```python
from build123d import *

# Parameters (mm, degrees)
BOSS_EXTRUDE1_DEPTH                   = 5
TAP_DRILL_FOR_M5X0_8_TAP1_D           = 4.2
TAP_DRILL_FOR_M5X0_8_TAP1_CSINK_D     = 4.25
TAP_DRILL_FOR_M5X0_8_TAP1_CSINK_ANGLE = 90
SKETCH4_W                             = 5
SKETCH4_H                             = 15
SKETCH4_H_2                           = 5
SKETCH4_W_2                           = 15
BOSS_EXTRUDE2_DEPTH                   = 15
TAP_DRILL_FOR_M5X0_8_TAP2_D           = 4.2
TAP_DRILL_FOR_M5X0_8_TAP2_CSINK_D     = 4.25
TAP_DRILL_FOR_M5X0_8_TAP2_CSINK_ANGLE = 90
TAP_DRILL_FOR_M5X0_8_TAP3_D           = 4.2
TAP_DRILL_FOR_M5X0_8_TAP3_CSINK_D     = 4.25
TAP_DRILL_FOR_M5X0_8_TAP3_CSINK_ANGLE = 90
CHAMFER1_SIZE                         = 5


with BuildPart() as part:
    # Sketch1 → Boss-Extrude1 (new body)
    with BuildSketch(Plane(origin=(0, 0, 0), x_dir=(1, 0, 0), z_dir=(0, 1, 0))):
        Polygon((9.5, 0), (20, 0), (20, 20), (0, 20), (0, 0), align=None)
    extrude(amount=BOSS_EXTRUDE1_DEPTH)

    # Tap Drill for M5x0.8 Tap1 (through all)
    with Locations(Plane(origin=(0, 0, 0), x_dir=(-1, 0, 0), z_dir=(0, -1, 0))):
        with Locations((-9.5, 10.5)):
            CounterSinkHole(TAP_DRILL_FOR_M5X0_8_TAP1_D / 2, TAP_DRILL_FOR_M5X0_8_TAP1_CSINK_D / 2, counter_sink_angle=TAP_DRILL_FOR_M5X0_8_TAP1_CSINK_ANGLE)

    # Sketch4 → Boss-Extrude2 (add)
    with BuildSketch(Plane(origin=(0, 5, 0), x_dir=(1, 0, 0), z_dir=(0, 1, 0))):
        with Locations((17.5, 12.5)):
            Rectangle(SKETCH4_W, SKETCH4_H)
        with Locations((17.5, 2.5)):
            Rectangle(SKETCH4_W, SKETCH4_H_2)
        with Locations((7.5, 2.5)):
            Rectangle(SKETCH4_W_2, SKETCH4_H_2)
    extrude(amount=BOSS_EXTRUDE2_DEPTH)

    # Tap Drill for M5x0.8 Tap2 (through all)
    with Locations(Plane.XY):
        with Locations((9.5, 10.5)):
            CounterSinkHole(TAP_DRILL_FOR_M5X0_8_TAP2_D / 2, TAP_DRILL_FOR_M5X0_8_TAP2_CSINK_D / 2, counter_sink_angle=TAP_DRILL_FOR_M5X0_8_TAP2_CSINK_ANGLE)

    # Tap Drill for M5x0.8 Tap3 (through all)
    with Locations(Plane(origin=(20, 0, 0), x_dir=(0, 0, -1), z_dir=(1, 0, 0))):
        with Locations((10.5, 10.5)):
            CounterSinkHole(TAP_DRILL_FOR_M5X0_8_TAP3_D / 2, TAP_DRILL_FOR_M5X0_8_TAP3_CSINK_D / 2, counter_sink_angle=TAP_DRILL_FOR_M5X0_8_TAP3_CSINK_ANGLE)

    # Chamfer1
    chamfer1_edges = [part.edges().sort_by_distance(p)[0] for p in [
        (0, 20, -2.5),
        (17.5, 20, -20),
        (0, 2.5, -20),
    ]]
    chamfer(chamfer1_edges, length=CHAMFER1_SIZE)


solid = part.part
```
The listing builds one solid part. Answer for the finished solid, in the listing's coordinates (mm). A direction names the side the tool comes from. Give positions to 0.01 mm unless a question says otherwise; leave off trailing zeros. Write each loop counter-clockwise with the first axis right and the second up, starting at its lowest first coordinate (ties: lowest second). Pieces come first, ordered by that corner, then holes. Notation, with made-up numbers: (77, 75.25) -> (132, 75.25) arc R25 cw to (132, 89.25) -> close; hole circle Ø4 at (23.25, -24). An arc over 180 degrees is marked (long way). Use one line per item in the form item = value.
1) Each of these flat-tipped pins is pushed along its axis until it touches: P1, Ø1.5, axis at y = 15.5, z = -6.5, coming from the -X side; P2, Ø5, axis at x = 12, y = 16.5, coming from the -Z side; P3, Ø12, axis at y = 11, z = -8.5, coming from the +X side; P4, Ø5.5, axis at x = 9.5, z = -10.5, coming from the +Y side. Where does it stop, or does it pass through?
Result:
P1 = 15
P2 = -5
P3 = 20
P4 = 5
2) Section B-B on z = -10.5 is taken. Write down the section's boundary in (x, y) (3 decimals), plus the area to 3 significant figures.
Result:
outline = (0, 0) -> (7.375, 0) -> (7.4, 0.025) -> (7.4, 5) -> (0, 5) -> close; (11.6, 0.025) -> (11.625, 0) -> (20, 0) -> (20, 8.375) -> (19.975, 8.4) -> (15, 8.4) -> (15, 5) -> (11.6, 5) -> close; (15, 12.6) -> (19.975, 12.6) -> (20, 12.625) -> (20, 20) -> (15, 20) -> close
area = 133 mm²
3) Section C-C on y = 3.5 is taken. Write down the section's boundary in (x, z), plus the area to 3 significant figures.
Result:
outline = (0, -15) -> (5, -20) -> (20, -20) -> (20, 0) -> (0, 0) -> close; hole circle Ø4.2 at (9.5, -10.5)
area = 374 mm²
4) For a pull along X with two mould halves and no side action, classify faces 3 (the flat face through (16, 20, -6)), 4 (the flat face through (15, 12, -13)), 5 (the cylindrical face through (7.4, 2.55, -10.59)) as +X half, -X half, draft (parallel to the pull), parting line (faces both ways), or undercut.
Result:
face_3 = draft
face_4 = -X half
face_5 = undercut
5) Section D-D on y = 17.25 is taken. Write down the section's boundary in (x, z), plus the area to 4 significant figures.
Result:
outline = (2.25, -5) -> (15, -5) -> (15, -17.75) -> (20, -17.75) -> (20, 0) -> (2.25, 0) -> close
area = 152.5 mm²
6) A tool of negligible diameter and unlimited length cuts with its end or side. For faces 1 (the cylindrical face through (17.45, 10.59, -12.6)), 2 (the flat face through (7, 5, -13)), from which of +Z, -Z, +X, -X, +Y, -Y can it reach the whole face along a straight path? Write none if from no direction.
Result:
face_1 = +X, -X
face_2 = -Z, -X, +Y
7) Straight lines are drawn through the part: probe 1 along Y at (x, z) = (9.5, -2.7); probe 2 along X at (y, z) = (1.2, -10.5); probe 3 along Z at (x, y) = (17.05, 10.5). For each, find the intervals that lie inside material, in ascending order.
Result:
probe_1 = 0 to 8.4, 12.6 to 20
probe_2 = 0 to 7.4, 11.6 to 20
probe_3 = -20 to -12.6, -8.4 to 0
8) Section A-A on x = 9.5 is taken. Write down the section's boundary in (y, z) (3 decimals).
Result:
outline = (0, -20) -> (5, -20) -> (5, -12.6) -> (0.025, -12.6) -> (0, -12.625) -> close; (0, -8.375) -> (0.025, -8.4) -> (5, -8.4) -> (5, -5) -> (8.4, -5) -> (8.4, -0.025) -> (8.375, 0) -> (0, 0) -> close; (12.6, -5) -> (20, -5) -> (20, 0) -> (12.625, 0) -> (12.6, -0.025) -> close
